Autodesk Inventor part; units mm, degrees
ref_plane "YZ Plane" through (0, 0, 0) normal (1, 0, 0) x (0, 1, 0)
ref_plane "XZ Plane" through (0, 0, 0) normal (0, 1, 0) x (-1, 0, 0)
ref_plane "XY Plane" through (0, 0, 0) normal (0, 0, 1) x (1, 0, 0)
sketch "Schizzo1" plane through (0, 0, 0) normal (0, 1, 0) x (-1, 0, 0)
  line L0 (9.5, 40) -> (-9.5, 40)
  line L1 (-9.5, 40) -> (-9.5, -40)
  line L2 (-9.5, -40) -> (9.5, -40)
  line L3 (9.5, -40) -> (9.5, 40)
  line L4 (9.5, 40) -> (-9.5, -40) construction
  line L5 (-9.5, 40) -> (9.5, -40) construction
  point P0 (0, 0)
  point P1 (0, 0)
  point P2 (0, 0)
  dimension "d0" = 19
  dimension "d15" = 80
extrude "Estrusione1" add sketch "Schizzo1" along normal blind 16
sketch "Schizzo2" plane through (0, 0, 0) normal (0, -1, 0) x (1, 0, 0)
  line L0 (9.5, 40) -> (9.5, -40)
  line L1 (9.5, 0) -> (10.5, 0)
  line L2 (9.5, 0) -> (10.5, 0) construction
  circle A0 centre (10.5, 0) radius 9.5
  point P0 (0, 0)
  dimension "d9" = 1
  dimension "d10" = 0
  dimension "d11" = 19
extrude "Estrusione2" cut sketch "Schizzo2" against normal blind 4
sketch "Schizzo4" plane through (0, 4, 0) normal (0, -1, 0) x (1, 0, 0)
  line L0 (9.5, 9.4472) -> (9.5, -9.4472)
  line L1 (9.5, 0) -> (10.5, 0)
  line L2 (9.5, 0) -> (10.5, 0) construction
  circle A0 centre (10.5, 0) radius 6
  point P0 (0, 0)
  point P1 (24.5, 9.5)
  point P2 (24.5, -9.5)
  dimension "d12" = 1
  dimension "d13" = 0
  dimension "d14" = 12
extrude "Estrusione3" cut sketch "Schizzo4" against normal blind 26
sketch "Schizzo8" plane through (0, 16, 0) normal (0, 1, 0) x (1, 0, 0)
  arc A0 (9.5, 5.9161) -> (9.5, -5.9161) centre (10.5, 0) ccw
  circle A1 centre (10.5, 0) radius 20
  line L0 (-9.5, 40) -> (-9.5, -40)
  line L1 (-9.5, 0) -> (-9.5, -40)
  line L2 (-9.5, -40) -> (0, -40)
  line L3 (-9.5, -40) -> (9.5, -40)
  line L4 (0, -40) -> (0, -17.022)
  line L5 (9.5, 40) -> (-9.5, 40)
  line L6 (-9.5, 0) -> (-9.5, 40)
  line L7 (-9.5, 40) -> (0, 40)
  line L8 (0, 40) -> (0, 17.022)
  point P0 (0, 0)
  dimension "d17" = 40
extrude "Estrusione4" cut sketch "Schizzo8" against normal blind 16 contours A1 L0 L5 L8 | L4 L2 L0 A1
sketch "Schizzo9" plane through (0, 16, -40) normal (-1, 0, 0) x (0, 0, 1)
  line L0 (40, -16) -> (40, -8)
  line L1 (40, -16) -> (48, -16) construction
  line L2 (40, -8) -> (15, -8)
  line L3 (40, -8) -> (65, -8)
  line L4 (40, -8) -> (65, -8) construction
  dimension "d20" = 8
  dimension "d21" = 90
  dimension "d22" = 25
  dimension "d23" = 90
  dimension "d24" = 25
  dimension "d25" = 0
hole "Foro1" at (0, 8, 25) at (0, 8, -25) direction (1, 0, 0) diameter 6.6 end through all
properties part number "15_Base_Dietro"
The listing builds one solid part. Answer for the finished solid, in the listing's coordinates (mm). A direction names the side the tool comes from. Round coordinates to 2 decimals unless told otherwise and drop trailing zeros. Write each loop counter-clockwise with the first axis right and the second up, starting at its lowest first coordinate (ties: lowest second). Pieces come first, ordered by that corner, then holes. Notation, with made-up numbers: (39, -36) - (56, -36) arc R14 ccw to (56, -13) - close; hole circle Ø2 at (2.5, 23). An arc over 180 degrees is marked (long way). Use one line per item in the form item = value. Start each with the question number.
Item 1: Find the intervals of material crossed by line 1 (Z direction, x = 4, y = 8); line 2 (Z direction, x = 7.75, y = 8); line 3 (Y direction, x = 7.75, z = 25), in increasing order. Write a range as [from, to].
Item 2: A cutting plane is placed at D-D (z = -24). Write down the section's boundary in (x, y).
Item 3: A cutting plane is placed at B-B (y = 8). Write down the section's boundary in (x, z).
Item 4: Flat-ended cylindrical pins translate along their axes: pin 1 Ø4 at (y, z) = (8, -25) entering from +X; pin 2 Ø6 at (y, z) = (11.5, 8.5) entering from -X; pin 3 Ø8 at (y, z) = (14, -24.5) entering from -X. Find the tip coordinate at first contact, or state that the pin passes through.
Item 5: Determine the mould class of faces 4 (the flat face through (5, 8, 40)), 5 (the flat face through (0, 8, 29)), 6 (the cylindrical face through (4.82, 9.26, -21.95)) for opening direction Z: +Z half, -Z half, draft (parallel to the pull), parting line (faces both ways), or undercut.
Item 6: A cutting plane is placed at A-A (z = 25). Write down the section's boundary in (x, y).
Item 7: A cutting plane is placed at C-C (x = 1.75). Write down the section's boundary in (y, z), plus the area to 3 significant figures.
Item 8: A tool of negligible diameter and unlimited length cuts with its end or side. For faces 1 (the flat face through (9.5, 11, 23)), 2 (the flat face through (0, 8, -29)), 3 (the flat face through (4, 4, 0)), from which of +Z, -Z, +X, -X, +Y, -Y can it reach the whole face along a straight path? Write none if from no direction.
The answers:
q1.line_1 = [-40, -28.3], [-21.7, 21.7], [28.3, 40]
q1.line_2 = [-40, -28.3], [-21.7, -5.33], [5.33, 21.7], [28.3, 40]
q1.line_3 = [0, 4.7], [11.3, 16]
q2.outline = (0, 0) - (9.5, 0) - (9.5, 4.86) - (0, 4.86) - close; (0, 11.14) - (9.5, 11.14) - (9.5, 16) - (0, 16) - close
q3.outline = (0, -40) - (9.5, -40) - (9.5, -28.3) - (0, -28.3) - close; (0, -21.7) - (9.5, -21.7) - (9.5, -5.92) arc R6 cw to (9.5, 5.92) - (9.5, 21.7) - (0, 21.7) - (0, 17.02) arc R20 ccw to (0, -17.02) - close; (0, 28.3) - (9.5, 28.3) - (9.5, 40) - (0, 40) - close
q4.pin_1 = through
q4.pin_2 = -8.73
q4.pin_3 = 0
q5.face_4 = +Z half
q5.face_5 = draft
q5.face_6 = undercut
q6.outline = (0, 0) - (9.5, 0) - (9.5, 4.7) - (0, 4.7) - close; (0, 11.3) - (9.5, 11.3) - (9.5, 16) - (0, 16) - close
q7.outline = (0, -40) - (16, -40) - (16, 40) - (0, 40) - (0, 3.7) - (4, 3.7) - (4, -3.7) - (0, -3.7) - close; hole circle Ø6.6 at (8, -25); hole circle Ø6.6 at (8, 25)
q7.area = 1,180 mm^2
q8.face_1 = +Z, -Z, +X, +Y, -Y
q8.face_2 = -Z, -X, +Y, -Y
q8.face_3 = +X, -Y
